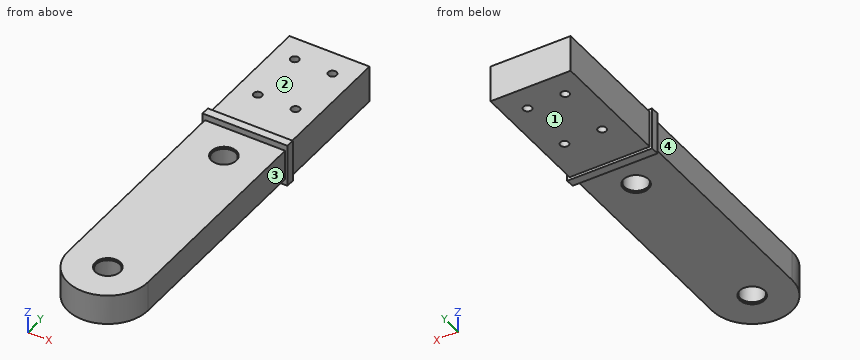
```python
from build123d import *

# Parameters (mm, degrees)
SKETCH1_R           = 7
SKETCH1_R_2         = 2.5
BOSS_EXTRUDE1_DEPTH = 9
SKETCH3_W           = 47.85
SKETCH3_H           = 65
SKETCH3_R           = 2.5
BOSS_EXTRUDE2_DEPTH = 11.025
SKETCH4_R           = 7.5
CUT_EXTRUDE1_DEPTH  = 1
CUT_EXTRUDE2_START  = -1
SKETCH5_R           = 7.5
CUT_EXTRUDE2_DEPTH  = 1
SKETCH6_R           = 7.5
CUT_EXTRUDE3_DEPTH  = 1
CUT_EXTRUDE4_START  = -1
SKETCH7_R           = 7.5
CUT_EXTRUDE4_DEPTH  = 1
BOSS_EXTRUDE3_START = 10
SKETCH8_W           = 50.8
SKETCH8_H           = 25.4
BOSS_EXTRUDE3_DEPTH = 5
SKETCH9_W           = 47.85
SKETCH9_H           = 22.05
BOSS_EXTRUDE4_DEPTH = 10


with BuildPart() as part:
    # Sketch1 → Boss-Extrude1 (new, symmetric)
    with BuildSketch(Plane.XY):
        with BuildLine():
            Line((-23.925, 0), (-23.925, 100))
            Line((-23.925, 100), (23.925, 100))
            Line((23.925, 100), (23.925, 0))
            Line((23.925, 0), (23.925, -110))
            ThreePointArc((23.925, -110), (16.91752974, -126.91752974), (0, -133.925))
            ThreePointArc((0, -133.925), (-16.91752974, -126.91752974), (-23.925, -110))
            Line((-23.925, -110), (-23.925, 0))
        make_face()
        Circle(SKETCH1_R, mode=Mode.SUBTRACT)
        with Locations((-11.25, 85)):
            Circle(SKETCH1_R_2, mode=Mode.SUBTRACT)
        with Locations((11.25, 85)):
            Circle(SKETCH1_R_2, mode=Mode.SUBTRACT)
        with Locations((11.25, 50)):
            Circle(SKETCH1_R_2, mode=Mode.SUBTRACT)
        with Locations((-11.25, 50)):
            Circle(SKETCH1_R_2, mode=Mode.SUBTRACT)
        with Locations((0, -110)):
            Circle(SKETCH1_R, mode=Mode.SUBTRACT)
    extrude(amount=BOSS_EXTRUDE1_DEPTH, both=True)

    # Sketch3 → Boss-Extrude2 (add, symmetric)
    with BuildSketch(Plane.XY):
        with Locations((0, 67.5)):
            Rectangle(SKETCH3_W, SKETCH3_H)
        with Locations((-11.25, 50)):
            Circle(SKETCH3_R, mode=Mode.SUBTRACT)
        with Locations((11.25, 50)):
            Circle(SKETCH3_R, mode=Mode.SUBTRACT)
        with Locations((11.25, 85)):
            Circle(SKETCH3_R, mode=Mode.SUBTRACT)
        with Locations((-11.25, 85)):
            Circle(SKETCH3_R, mode=Mode.SUBTRACT)
    extrude(amount=BOSS_EXTRUDE2_DEPTH, both=True)

    # Sketch4 → Cut-Extrude1 (cut)
    with BuildSketch(Plane.XY.offset(9)):
        with Locations((0, -110)):
            Circle(SKETCH4_R)
    extrude(amount=-CUT_EXTRUDE1_DEPTH, mode=Mode.SUBTRACT)

    # Sketch5 → Cut-Extrude2 (cut)
    with BuildSketch(Plane(origin=(0, 0, -9), x_dir=(-1, 0, 0), z_dir=(0, 0, -1)).offset(CUT_EXTRUDE2_START)):
        with Locations(Location((0, -110, 0), (0, 0, 180))):
            Circle(SKETCH5_R)
    extrude(amount=CUT_EXTRUDE2_DEPTH, mode=Mode.SUBTRACT)

    # Sketch6 → Cut-Extrude3 (cut)
    with BuildSketch(Plane.XY.offset(9)):
        Circle(SKETCH6_R)
    extrude(amount=-CUT_EXTRUDE3_DEPTH, mode=Mode.SUBTRACT)

    # Sketch7 → Cut-Extrude4 (cut)
    with BuildSketch(Plane(origin=(0, 0, -9), x_dir=(-1, 0, 0), z_dir=(0, 0, -1)).offset(CUT_EXTRUDE4_START)):
        with Locations(Location((0, 0, 0), (0, 0, 180))):
            Circle(SKETCH7_R)
    extrude(amount=CUT_EXTRUDE4_DEPTH, mode=Mode.SUBTRACT)

    # Sketch8 → Boss-Extrude3 (add)
    with BuildSketch(Plane.XZ.offset(-35).offset(BOSS_EXTRUDE3_START)):
        Rectangle(SKETCH8_W, SKETCH8_H)
    extrude(amount=BOSS_EXTRUDE3_DEPTH)

    # Sketch9 → Boss-Extrude4 (add)
    with BuildSketch(Plane.XZ.offset(-35)):
        Rectangle(SKETCH9_W, SKETCH9_H)
    extrude(amount=BOSS_EXTRUDE4_DEPTH)


solid = part.part
```
Source: CAD feature listing. Evaluate the final solid. Frame: model axes, mm. Face numbers are marked on the shaded views. A direction names the side the tool comes from. Give positions to 0.01 mm unless a question says otherwise; leave off trailing zeros. Write each loop counter-clockwise with the first axis right and the second up, starting at its lowest first coordinate (ties: lowest second). Pieces come first, ordered by that corner, then holes. Notation, with made-up numbers: (65, 86) - (109, 86) arc R4 ccw to (109, 91) - close; hole circle Ø11 at (55.5, 52.5). An arc over 180 degrees is marked (long way). One line per item, written item: value. Start each with the question number.
Q1. Section query B-B, the plane z = 3.5. Return the cut outline in (x, y) (3 decimals).
Q2. Material intervals for probe 1 along Y at (x, z) = (0, 1.25) (3 decimals); probe 2 along Y at (x, z) = (0, 8.4) (3 decimals); probe 3 along X at (y, z) = (0, 3) (3 decimals), sorted ascending. Write a range as from..to.
Q3. Set-up query: the marked faces 1, 2, 3 and 4. Return all of +Z, -Z, +X, -X, +Y, -Y with unobstructed straight access to the full face (end or side cutting, diameter ignored); none if empty.
Q4. Section query C-C, the plane x = -20. Return the cut outline in (y, z) (3 decimals).
Q5. Section query A-A, the plane y = 0. Return the cut outline in (x, z) (3 decimals), then the cut area to 3 significant figures.
Q6. First-contact query: pin 1 Ø16.5 at (x, y) = (0.5, -3) entering from -Z; pin 2 Ø2 at (x, z) = (14, 4) entering from -Y; pin 3 Ø7.5 at (x, y) = (3.5, 1) entering from +Z. Flat tips, straight axial feed; report the tip coordinate or a pass-through.
Q7. Section query D-D, the plane x = 0. Count the separate pieces of the cut face and the enclosed holes in it, then the cut area to 3 significant figures.
Answer:
1. outline: (-25.4, 20) - (-23.925, 20) - (-23.925, -110) arc R23.925 ccw to (23.925, -110) - (23.925, 20) - (25.4, 20) - (25.4, 25) - (23.925, 25) - (23.925, 100) - (-23.925, 100) - (-23.925, 25) - (-25.4, 25) - close; hole circle Ø5 at (-11.25, 50); hole circle Ø5 at (-11.25, 85); hole circle Ø14 at (0, -110); hole circle Ø14 at (0, 0); hole circle Ø5 at (11.25, 50); hole circle Ø5 at (11.25, 85)
2. probe 1: y = -133.925..-117, -103..-7, 7..100
2. probe 2: y = -133.925..-117.5, -102.5..-7.5, 7.5..100
2. probe 3: x = -23.925..-7, 7..23.925
3. face 1: -Z, +X, -X, +Y
3. face 2: +Z, +X, -X, +Y
3. face 3: +Z, -Z, +X, -Y
3. face 4: +Z, -Z, -X, -Y
4. outline: (-123.13, -9) - (20, -9) - (20, -12.7) - (25, -12.7) - (25, -11.025) - (100, -11.025) - (100, 11.025) - (25, 11.025) - (25, 12.7) - (20, 12.7) - (20, 9) - (-123.13, 9) - close
5. outline: (-23.925, -9) - (-7.5, -9) - (-7.5, -8) - (-7, -8) - (-7, 8) - (-7.5, 8) - (-7.5, 9) - (-23.925, 9) - close; (7, -8) - (7.5, -8) - (7.5, -9) - (23.925, -9) - (23.925, 9) - (7.5, 9) - (7.5, 8) - (7, 8) - close
5. area: 607 mm2
6. pin 1: stops at z = -9
6. pin 2: stops at y = -130.08
6. pin 3: stops at z = 8
7. separate pieces: 3
7. enclosed holes: 0
7. area: 4,040 mm2
